Geometry check sheet. Reference: the model listing, model coordinates, mm. Face numbers are marked on the shaded views. A direction names the side the tool comes from. Coordinates: 2 decimals unless noted, no trailing zeros. Order: outer loops, then holes, each group sorted by start corner. A loop starts at its lowest first (then second) coordinate and runs counter-clockwise, first axis right, second up.
```python
from build123d import *

# Parameters (mm, degrees)
SKETCH_4_R          = 2.5
EXTRUDE_3_DEPTH     = 25
SKETCH_5_R          = 7.5
EXTRUDE_4_DEPTH     = 25
SKETCH_6_R          = 139.999706489
EXTRUDE_5_DEPTH     = 19
SKETCH_15_W         = 120
SKETCH_15_H         = 27.7
EXTRUDE_7_DEPTH     = 100
CUT_EXTRUDE_3_REACH = 309.363
SKETCH_16_R         = 30
CUT_EXTRUDE_4_REACH = 309.363
SKETCH_17_R         = 30
SKETCH_18_R         = 2
EXTRUDE_8_DEPTH     = 30
SKETCH_19_R         = 5
CUT_EXTRUDE_5_DEPTH = 222.810359618


with BuildPart() as part:
    # 草图4 → 凸台-拉伸3 (new body)
    with BuildSketch(Plane(origin=(0, 0, 0), x_dir=(1, 0, 0), z_dir=(0, 1, 0))):
        with Locations(Location((0, 0, 0), (0, 0, 270))):
            Circle(SKETCH_4_R)
    extrude(amount=EXTRUDE_3_DEPTH)

    # 草图5 → 凸台-拉伸4 (add)
    with BuildSketch(Plane(origin=(0, 25, 0), x_dir=(1, 0, 0), z_dir=(0, 1, 0))):
        with Locations(Location((0, 0, 0), (0, 0, 270))):
            Circle(SKETCH_5_R)
    extrude(amount=EXTRUDE_4_DEPTH)

    # 草图6 → 凸台-拉伸5 (add)
    with BuildSketch(Plane(origin=(0, 50, 0), x_dir=(1, 0, 0), z_dir=(0, 1, 0))):
        with Locations(Location((0, 0, 0), (0, 0, 270))):
            Circle(SKETCH_6_R)
    extrude(amount=-EXTRUDE_5_DEPTH)

    # 草图15 → 凸台-拉伸7 (add)
    with BuildSketch(Plane(origin=(0, 50, 0), x_dir=(1, 0, 0), z_dir=(0, 1, 0))):
        with Locations((0, 75)):
            Rectangle(SKETCH_15_W, SKETCH_15_H)
        with Locations((0, -75)):
            Rectangle(SKETCH_15_W, SKETCH_15_H)
    extrude(amount=EXTRUDE_7_DEPTH)

    # 草图16 → 切除-拉伸3 (cut, up to next)
    with BuildSketch(Plane.XY.offset(88.85), mode=Mode.PRIVATE) as cut_extrude_3_sk1:
        with Locations((0, 100)):
            Circle(SKETCH_16_R)
    cut_extrude_3_tool1 = extrude(cut_extrude_3_sk1.sketch, amount=-CUT_EXTRUDE_3_REACH, mode=Mode.PRIVATE) & part.part
    add(cut_extrude_3_tool1.solids().sort_by_distance((0, 100, 88.85))[0], mode=Mode.SUBTRACT)

    # 草图17 → 切除-拉伸4 (cut, up to next)
    with BuildSketch(Plane(origin=(0, 0, -88.85), x_dir=(-1, 0, 0), z_dir=(0, 0, -1)), mode=Mode.PRIVATE) as cut_extrude_4_sk1:
        with Locations(Location((0, 100, 0), (0, 0, 180))):
            Circle(SKETCH_17_R)
    cut_extrude_4_tool1 = extrude(cut_extrude_4_sk1.sketch, amount=-CUT_EXTRUDE_4_REACH, mode=Mode.PRIVATE) & part.part
    add(cut_extrude_4_tool1.solids().sort_by_distance((0, 100, -88.85))[0], mode=Mode.SUBTRACT)

    # 草图18 → 凸台-拉伸8 (add)
    with BuildSketch(Plane.XZ.offset(-31)):
        with Locations(Location((0, 17.25, 0), (0, 0, 90))):
            Circle(SKETCH_18_R)
        with Locations(Location((14.938938215, 8.625, 0), (0, 0, 90))):
            Circle(SKETCH_18_R)
        with Locations(Location((14.938938215, -8.625, 0), (0, 0, 90))):
            Circle(SKETCH_18_R)
        with Locations(Location((0, -17.25, 0), (0, 0, 90))):
            Circle(SKETCH_18_R)
        with Locations(Location((-14.938938215, -8.625, 0), (0, 0, 90))):
            Circle(SKETCH_18_R)
        with Locations(Location((-14.938938215, 8.625, 0), (0, 0, 90))):
            Circle(SKETCH_18_R)
    extrude(amount=EXTRUDE_8_DEPTH)

    # 草图19 → 切除-拉伸5 (cut, symmetric)
    with BuildSketch(Plane(origin=(0, 50, 0), x_dir=(1, 0, 0), z_dir=(0, 1, 0))):
        with Locations(Location((108.378245134, 0, 0), (0, 0, 270))):
            Circle(SKETCH_19_R)
    cut_extrude_5 = extrude(amount=CUT_EXTRUDE_5_DEPTH, both=True, mode=Mode.SUBTRACT)

    # 镜向1: 切除-拉伸5 across plane
    add(cut_extrude_5.mirror(Plane(origin=(0, 0, 0), x_dir=(0, 0, 1), z_dir=(1, 0, 0))), mode=Mode.SUBTRACT)


solid = part.part
```
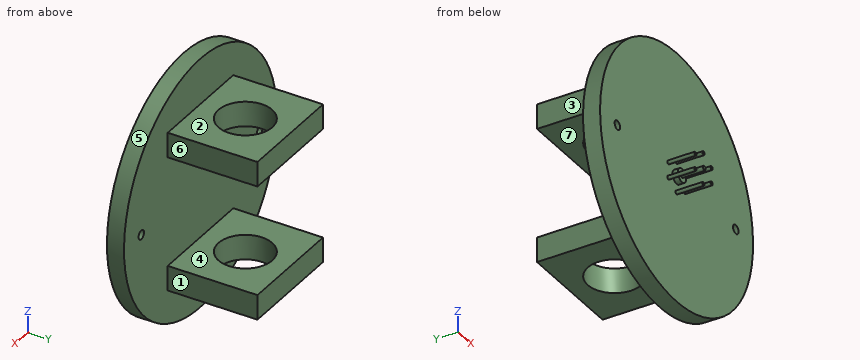
Item 1: Release check for a two-part mould opening along Z. For the marked faces 4, 5, 6 and 7 record: pulls with the +Z half, pulls with the -Z half, needs draft (parallel to the pull), parting line crosses it, or undercut.
Item 2: Depth check by flat-ended pin: P1, Ø12, axis at x = -82.5, y = 53.5, coming from the +Z side; P2, Ø5, axis at x = -56, y = 33, coming from the -Z side; P3, Ø2, axis at x = -15, z = 7.5, coming from the -Y side; P4, Ø12, axis at y = 21.5, z = 74.5, coming from the +X side. Enter the tip coordinate at first touch or a pass-through.
Item 3: Tool access check on the marked faces 1, 2 and 3. Record the directions out of +Z, -Z, +X, -X, +Y, -Y that give a thin tool (end or side, any length) a straight path to the whole face; none if there is none.
Item 4: Sectioned sample at A-A (y = 100). Record the cut outline in (x, z).
Item 5: Thickness scan on line 1 along Y through (x, z) = (0, -76.25); line 2 along Z through (x, y) = (-57.5, 130); line 3 along X through (y, z) = (35.5, 0). Record the ranges inside material, lowest first.
Item 6: Sectioned sample at D-D (y = 124.5). Record the cut outline in (x, z), and give its area (3 significant figures).
Item 7: Sectioned sample at B-B (z = -77). Record the cut outline in (x, y), and give its area (3 significant figures).
Item 8: Sectioned sample at C-C (x = -47). Record the cut outline in (y, z).
Geometry check:
1. face 4: undercut
1. face 5: parting line crosses it
1. face 6: needs draft
1. face 7: undercut
2. P1: stops at z = 116.51
2. P2: stops at z = -129.37
2. P3: stops at y = 1
2. P4: passes through
3. face 1: +Z, -Z, +X, +Y
3. face 2: +Z, +X, -X, +Y
3. face 3: +Z, -Z, -X, +Y
4. outline: (-60, -88.85) - (-30, -88.85) - (-30, -61.15) - (-60, -61.15) - close; (-60, 61.15) - (-30, 61.15) - (-30, 88.85) - (-60, 88.85) - close; (30, -88.85) - (60, -88.85) - (60, -61.15) - (30, -61.15) - close; (30, 61.15) - (60, 61.15) - (60, 88.85) - (30, 88.85) - close
5. line 1: y = 31 to 70, 130 to 150
5. line 2: z = -88.85 to -61.15, 61.15 to 88.85
5. line 3: x = -140 to -113.38, -103.38 to 103.38, 113.38 to 140
6. outline: (-60, -88.85) - (-17.31, -88.85) - (-17.31, -61.15) - (-60, -61.15) - close; (-60, 61.15) - (-17.31, 61.15) - (-17.31, 88.85) - (-60, 88.85) - close; (17.31, -88.85) - (60, -88.85) - (60, -61.15) - (17.31, -61.15) - close; (17.31, 61.15) - (60, 61.15) - (60, 88.85) - (17.31, 88.85) - close
6. area: 4,730 mm2
7. outline: (-116.92, 31) - (116.92, 31) - (116.92, 50) - (60, 50) - (60, 150) - (-60, 150) - (-60, 50) - (-116.92, 50) - close; hole circle Ø60 at (0, 100)
7. area: 13,600 mm2
8. outline: (31, -131.87) - (50, -131.87) - (50, -88.85) - (150, -88.85) - (150, -61.15) - (50, -61.15) - (50, 61.15) - (150, 61.15) - (150, 88.85) - (50, 88.85) - (50, 131.87) - (31, 131.87) - close
